The listing builds one solid part. Answer for the finished solid, in the listing's coordinates (mm). A direction names the side the tool comes from. Round coordinates to 2 decimals unless told otherwise and drop trailing zeros. Write each loop counter-clockwise with the first axis right and the second up, starting at its lowest first coordinate (ties: lowest second). Pieces come first, ordered by that corner, then holes.
Item 1: Find section C-C on y = -1.5. Give the vertices of the cut face in (x, z).
Item 2: Find the intervals of material crossed by probe 1 along Y at (x, z) = (8, 0.5); probe 2 along Y at (x, z) = (-9.5, -0.25); probe 3 along X at (y, z) = (4.5, 2.5), in increasing order.
Item 3: This flat-tipped pin is pushed along its axis until it touches: pin 1 (6 mm diameter, centred on x = 0, y = -2.5, fed in from -Z). Where does it stop, or does it pass through?
Item 4: A tool of negligible diameter and unlimited length cuts with its end or side. For faces 5 (the face through (4, 0, -2)), 6 (the face through (0, 0, 6.5)), from which of +Z, -Z, +X, -X, +Y, -Y can it reach the whole face along a straight path? Write none if from no direction.
Item 5: Find section A-A on z = -1.5. Give the vertices of the cut face in (x, y).
Item 6: For a pull along X with two mould halves and no side action, classify faces 1 (the face through (0, 9, 5)), 2 (the face through (-7.63, 3.34, 1.43)), 3 (the face through (-12, 0, 2)), 4 (the face through (-4, 0, -2)) as +X half, -X half, draft (parallel to the pull), parting line (faces both ways), or undercut.
Item 7: Find section B-B on x = -8. Give the vertices of the cut face in (y, z), then the cut area to 3 significant figures.
Item 8: Find section D-D on z = 4.5. Give the vertices of the cut face in (x, y).
```python
from build123d import *

# Parameters (mm, degrees)
SKETCH1_W           = 24
SKETCH1_H           = 18
BOSS_EXTRUDE1_DEPTH = 10
CUT_EXTRUDE1_DEPTH  = 23.588713996
HOLE1_D             = 3.4
HOLE2_D             = 3.4
HOLE3_D             = 3.4
HOLE4_D             = 3.4


with BuildPart() as part:
    # Sketch1 → Boss-Extrude1 (new body)
    with BuildSketch(Plane.XY.offset(6.5)):
        Rectangle(SKETCH1_W, SKETCH1_H)
    extrude(amount=-BOSS_EXTRUDE1_DEPTH)

    # Sketch2 → Cut-Extrude1 (cut, through all)
    with BuildSketch(Plane(origin=(0, 9, 0), x_dir=(-1, 0, 0), z_dir=(0, 1, 0))):
        with BuildLine():
            Line((-4, -3.5), (4, -3.5))
            Line((4, -3.5), (4, 0))
            ThreePointArc((4, 0), (0, 4), (-4, 0))
            Line((-4, 0), (-4, -3.5))
        make_face()
    extrude(amount=-CUT_EXTRUDE1_DEPTH, mode=Mode.SUBTRACT)

    # Hole1 (through all)
    with Locations(Plane.XY.offset(6.5)):
        with Locations((8, -5)):
            Hole(HOLE1_D / 2)

    # Hole2 (through all)
    with Locations(Plane.XY.offset(6.5)):
        with Locations((-8, 5)):
            Hole(HOLE2_D / 2)

    # Hole3 (through all)
    with Locations(Plane.XY.offset(6.5)):
        with Locations((-8, -5)):
            Hole(HOLE3_D / 2)

    # Hole4 (through all)
    with Locations(Plane.XY.offset(6.5)):
        with Locations((8, 5)):
            Hole(HOLE4_D / 2)


solid = part.part
```
Check values:
1. outline: (-12, -3.5) - (-4, -3.5) - (-4, 0) arc R4 cw to (4, 0) - (4, -3.5) - (12, -3.5) - (12, 6.5) - (-12, 6.5) - close
2. probe 1: y = -9 to -6.7, -3.3 to 3.3, 6.7 to 9
2. probe 2: y = -9 to -5.8, -4.2 to 4.2, 5.8 to 9
2. probe 3: x = -12 to -9.62, -6.38 to -3.12, 3.12 to 6.38, 9.62 to 12
3. pin 1: stops at z = 2.65
4. face 5: -Z, +Y, -Y
4. face 6: +Z, +X, -X, +Y, -Y
5. outline: (-12, -9) - (-4, -9) - (-4, 9) - (-12, 9) - close; (4, -9) - (12, -9) - (12, 9) - (4, 9) - close; hole circle Ø3.4 at (-8, -5); hole circle Ø3.4 at (-8, 5); hole circle Ø3.4 at (8, -5); hole circle Ø3.4 at (8, 5)
6. face 1: draft
6. face 2: undercut
6. face 3: -X half
6. face 4: undercut
7. outline: (-9, -3.5) - (-6.7, -3.5) - (-6.7, 6.5) - (-9, 6.5) - close; (-3.3, -3.5) - (3.3, -3.5) - (3.3, 6.5) - (-3.3, 6.5) - close; (6.7, -3.5) - (9, -3.5) - (9, 6.5) - (6.7, 6.5) - close
7. area: 112 mm2
8. outline: (-12, -9) - (12, -9) - (12, 9) - (-12, 9) - close; hole circle Ø3.4 at (-8, -5); hole circle Ø3.4 at (-8, 5); hole circle Ø3.4 at (8, -5); hole circle Ø3.4 at (8, 5)
